```python
from build123d import *

# Parameters (mm, degrees)
SKETCH1_R           = 31.5
SKETCH1_R_2         = 22.625
BOSS_EXTRUDE1_DEPTH = 1.5
SKETCH2_R           = 1.5
BOSS_EXTRUDE2_DEPTH = 3


with BuildPart() as part:
    # Sketch1 → Boss-Extrude1 (new body)
    with BuildSketch(Plane(origin=(0, 0, 0), x_dir=(1, 0, 0), z_dir=(0, 1, 0))):
        with Locations(Location((0, 0, 0), (0, 0, 270))):
            Circle(SKETCH1_R)
        with Locations(Location((0, 0, 0), (0, 0, 270))):
            Circle(SKETCH1_R_2, mode=Mode.SUBTRACT)
        with BuildLine():
            ThreePointArc((-11.821381939, 22.907790728), (-7.904609513, 27.531658188), (-2.147738601, 29.423666069))
            ThreePointArc((-2.147738601, 29.423666069), (-1.106349013, 28.466844389), (-2.063170693, 27.425454801))
            ThreePointArc((-2.063170693, 27.425454801), (-6.78729401, 25.872861616), (-10.001421306, 22.07848783))
            ThreePointArc((-10.001421306, 22.07848783), (-11.326053072, 21.583158963), (-11.821381939, 22.907790728))
        make_face(mode=Mode.SUBTRACT)
        with BuildLine():
            ThreePointArc((17.907280569, 16.334544855), (22.509164441, 14.450254128), (25.445602695, 10.437123544))
            ThreePointArc((25.445602695, 10.437123544), (26.731697208, 9.848939131), (27.319881621, 11.135033644))
            ThreePointArc((27.319881621, 11.135033644), (23.741504251, 16.02548065), (18.13359573, 18.321698963))
            ThreePointArc((18.13359573, 18.321698963), (17.026861096, 17.44127949), (17.907280569, 16.334544855))
        make_face(mode=Mode.SUBTRACT)
        with BuildLine():
            ThreePointArc((21.068729344, -11.983183919), (20.698722692, -16.942113419), (17.789418023, -20.974957706))
            ThreePointArc((17.789418023, -20.974957706), (17.627446465, -22.379865253), (19.032354011, -22.541836811))
            ThreePointArc((19.032354011, -22.541836811), (22.577666084, -17.62736646), (23.028560438, -11.584358037))
            ThreePointArc((23.028560438, -11.584358037), (21.849231951, -10.803855431), (21.068729344, -11.983183919))
        make_face(mode=Mode.SUBTRACT)
        with BuildLine():
            ThreePointArc((-4.886089735, -23.74055981), (-9.716650293, -24.921056063), (-14.451137717, -23.400360319))
            ThreePointArc((-14.451137717, -23.400360319), (-15.837336158, -23.680456521), (-15.557239956, -25.066654962))
            ThreePointArc((-15.557239956, -25.066654962), (-9.787739224, -26.919792254), (-3.901162667, -25.481225968))
            ThreePointArc((-3.901162667, -25.481225968), (-3.523293122, -24.118429356), (-4.886089735, -23.74055981))
        make_face(mode=Mode.SUBTRACT)
        with BuildLine():
            ThreePointArc((-24.088498872, -2.689288956), (-26.70394283, 1.540053737), (-26.720712308, 6.51273968))
            ThreePointArc((-26.720712308, 6.51273968), (-27.415458501, 7.744538254), (-28.647257075, 7.04979206))
            ThreePointArc((-28.647257075, 7.04979206), (-28.626821597, 0.990019877), (-25.439611562, -4.163905686))
            ThreePointArc((-25.439611562, -4.163905686), (-24.026746852, -4.102153666), (-24.088498872, -2.689288956))
        make_face(mode=Mode.SUBTRACT)
    extrude(amount=BOSS_EXTRUDE1_DEPTH)

    # Sketch2 → Boss-Extrude2 (add)
    with BuildSketch(Plane(origin=(0, 1.5, 0), x_dir=(1, 0, 0), z_dir=(0, 1, 0))):
        with Locations(Location((-21.264622422, 16.637783303, 0), (0, 0, 270))):
            Circle(SKETCH2_R)
        with Locations(Location((9.252342519, 25.365215511, 0), (0, 0, 270))):
            Circle(SKETCH2_R)
        with Locations(Location((26.982884575, -0.961217985, 0), (0, 0, 270))):
            Circle(SKETCH2_R)
        with Locations(Location((7.423997262, -25.959280896, 0), (0, 0, 270))):
            Circle(SKETCH2_R)
        with Locations(Location((-22.394601934, -15.082499932, 0), (0, 0, 270))):
            Circle(SKETCH2_R)
    extrude(amount=BOSS_EXTRUDE2_DEPTH)


solid = part.part
```
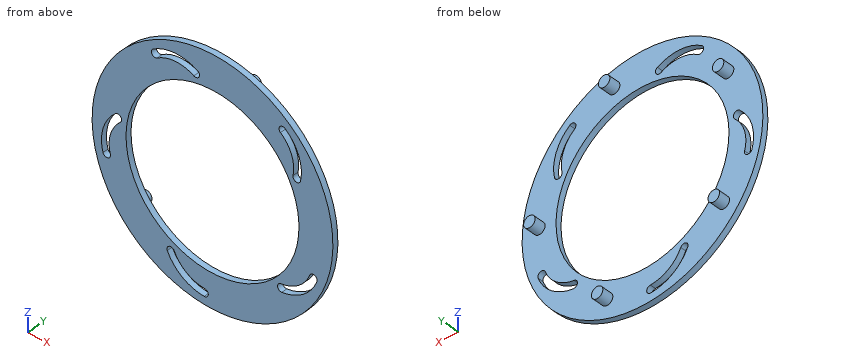
The listing builds one solid part. Answer for the finished solid, in the listing's coordinates (mm). Round coordinates to 2 decimals unless told otherwise and drop trailing zeros. Loops run counter-clockwise (first coordinate to the right, second up) from the corner with the lowest first, then second, coordinate; pieces in that order, holes last. Notation, with made-up numbers: (76, 23) -> (105, 23) arc R31 ccw to (105, 61) -> close; hole circle Ø2 at (28, 84). An arc over 180 degrees is marked (long way). Use one line per item in the form item = value.
1. The part is cut by section B-B on z = 18. Determine the outline of the cut face in (x, y).
Answer key:
outline = (-25.85, 0) -> (-13.71, 0) -> (-13.71, 1.5) -> (-25.85, 1.5) -> close; (13.71, 0) -> (20.24, 0) -> (20.24, 1.5) -> (13.71, 1.5) -> close; (22.43, 0) -> (25.85, 0) -> (25.85, 1.5) -> (22.43, 1.5) -> close
2. A flat-ended cylindrical pin translates along its axis: pin 1 Ø2 at (y, z) = (3.5, 14) entering from +X. Find the tip coordinate at first contact, or state that the pin passes through.
Answer key:
pin_1 = -20.9
3. The part is cut by section D-D on x = 24.5. Determine the outline of the cut face in (y, z).
Answer key:
outline = (0, -19.8) -> (1.5, -19.8) -> (1.5, -15.38) -> (0, -15.38) -> close; (0, -12.3) -> (1.5, -12.3) -> (1.5, 19.8) -> (0, 19.8) -> close
4. The part is cut by section A-A on x = 0. Determine the outline of the cut face in (y, z) (3 decimals).
Answer key:
outline = (0, -31.5) -> (1.5, -31.5) -> (1.5, -22.625) -> (0, -22.625) -> close; (0, 22.625) -> (1.5, 22.625) -> (1.5, 31.5) -> (0, 31.5) -> close
5. The part is cut by section C-C on y = 3.75. Determine the outline of the cut face in (x, z).
Answer key:
outline = circle Ø3 at (-22.39, 15.08); circle Ø3 at (-21.26, -16.64); circle Ø3 at (7.42, 25.96); circle Ø3 at (9.25, -25.37); circle Ø3 at (26.98, 0.96)
6. Find the intervals of material crossed by probe 1 along X at (y, z) = (0.55, 0) (3 decimals); probe 2 along X at (y, z) = (0.25, 20); probe 3 along X at (y, z) = (0.75, -26), in increasing order. Write a range as [from, to].
Answer key:
probe_1 = [-31.5, -28.293], [-26.108, -22.625], [22.625, 31.5]
probe_2 = [-24.34, -10.58], [10.58, 18.84], [21.37, 24.34]
probe_3 = [-17.78, -9.72], [-6.59, 17.78]
